CAD build for the part. Positions are in the model's coordinates, mm. Face numbers are marked on the shaded views. A direction names the side the tool comes from. Coordinates: 2 decimals unless noted, no trailing zeros. Write each loop counter-clockwise with the first axis right and the second up, starting at its lowest first coordinate (ties: lowest second). Pieces come first, ordered by that corner, then holes. Notation, with made-up numbers: (5, 69.5) -> (22, 69.5) arc R34 cw to (22, 106.5) -> close; hole circle Ø4 at (87, 17.25). An arc over 180 degrees is marked (long way). Answer as CSV lines item,"result". Start each with the question number.
```python
from build123d import *

# Parameters (mm, degrees)
SKETCH1_W                      = 114.3
SKETCH1_H                      = 139.7
BOSS_EXTRUDE1_DEPTH            = 31.836483884
SKETCH2_W                      = 109.4232
SKETCH2_H                      = 29.474283884
CUT_EXTRUDE1_DEPTH             = 203.397374705
M4_CLEARANCE_HOLE1_D           = 4.7625
M4_CLEARANCE_HOLE1_DEPTH       = 31.836483884
M3_CLEARANCE_HOLE1_D           = 3.59918
M2_CLEARANCE_HOLE1_D           = 2.286
M2_CLEARANCE_HOLE1_DEPTH       = 31.836483884
M4_CLEARANCE_HOLE2_D           = 4.7625
F_3_1_3_1_DIAMETER_HOLE1_D     = 3.1
M4_CLEARANCE_HOLE3_D           = 4.7625
M4_CLEARANCE_HOLE3_DEPTH       = 2.3622
F_3_1_3_1_DIAMETER_HOLE2_D     = 3.1
F_3_1_3_1_DIAMETER_HOLE2_DEPTH = 2.3622
FILLET1_R                      = 0.7366
FILLET2_R                      = 3.175


with BuildPart() as part:
    # Sketch1 → Boss-Extrude1 (new body)
    with BuildSketch(Plane.XZ.offset(31.836483884)):
        with Locations((85.8012, -50.8)):
            Rectangle(SKETCH1_W, SKETCH1_H)
    extrude(amount=-BOSS_EXTRUDE1_DEPTH)

    # Sketch2 → Cut-Extrude1 (cut, through all)
    with BuildSketch(Plane(origin=(0, 0, -120.65), x_dir=(-1, 0, 0), z_dir=(0, 0, -1))):
        with Locations((-85.725, -17.099341942)):
            Rectangle(SKETCH2_W, SKETCH2_H)
    extrude(amount=-CUT_EXTRUDE1_DEPTH, mode=Mode.SUBTRACT)

    # M4 Clearance Hole1
    with Locations(Plane(origin=(0, 0, 0), x_dir=(1, 0, 0), z_dir=(0, 1, 0))):
        with Locations((117.475, 95.25), (53.975, 51.246745007), (117.475, 51.246745007), (53.975, 95.25)):
            Hole(M4_CLEARANCE_HOLE1_D / 2, depth=M4_CLEARANCE_HOLE1_DEPTH)

    # M3 Clearance Hole1 (through all)
    with Locations(Plane(origin=(0, 0, 0), x_dir=(1, 0, 0), z_dir=(0, 1, 0))):
        with Locations((104.4702, -12.7), (53.74894, 28.51658), (105.08488, 33.24352), (53.91894, 1.777120394)):
            Hole(M3_CLEARANCE_HOLE1_D / 2)

    # M2 Clearance Hole1
    with Locations(Plane(origin=(0, 0, 0), x_dir=(1, 0, 0), z_dir=(0, 1, 0))):
        with Locations((92.456, 107.95), (78.994, 107.95), (78.994, -12.7), (92.456, -12.7)):
            Hole(M2_CLEARANCE_HOLE1_D / 2, depth=M2_CLEARANCE_HOLE1_DEPTH)

    # M4 Clearance Hole2 (through all)
    with Locations(Plane(origin=(142.9512, 0, 0), x_dir=(0, 0, -1), z_dir=(1, 0, 0))):
        with Locations((12.7, -19.136483884), (-12.7, -19.136483884), (0, -19.136483884), (88.9, -19.136483884), (101.6, -19.136483884), (114.3, -19.136483884)):
            Hole(M4_CLEARANCE_HOLE2_D / 2)

    # Ø3.1 (3.1) Diameter Hole1 (through all)
    with Locations(Plane(origin=(142.9512, 0, 0), x_dir=(0, 0, -1), z_dir=(1, 0, 0))):
        with Locations((47.09318, -27.181483884), (87.75, -27.181483884), (47.09318, -10.881483884), (87.77636, -10.881483884), (6.41, -10.881483884), (6.41, -27.181483884)):
            Hole(F_3_1_3_1_DIAMETER_HOLE1_D / 2)

    # M4 Clearance Hole3
    with Locations(Plane(origin=(31.0134, 0, 0), x_dir=(0, 0, -1), z_dir=(1, 0, 0))):
        with Locations((12.7, -19.136483884), (-12.7, -19.136483884), (0, -19.136483884)):
            Hole(M4_CLEARANCE_HOLE3_D / 2, depth=M4_CLEARANCE_HOLE3_DEPTH)

    # Ø3.1 (3.1) Diameter Hole2
    with Locations(Plane(origin=(31.0134, 0, 0), x_dir=(0, 0, -1), z_dir=(1, 0, 0))):
        with Locations((47.05, -27.181483884), (87.75, -27.181483884), (47.05, -10.881483884), (87.75, -10.881483884)):
            Hole(F_3_1_3_1_DIAMETER_HOLE2_D / 2, depth=F_3_1_3_1_DIAMETER_HOLE2_DEPTH)

    # Fillet1
    fillet1_edges = [part.edges().sort_by_distance(p)[0] for p in [
        (140.4366, -2.3622, -50.8),
        (31.0134, -2.3622, -50.8),
    ]]
    fillet(fillet1_edges, radius=FILLET1_R)

    # Fillet2
    fillet2_edges = [part.edges().sort_by_distance(p)[0] for p in [
        (28.6512, 0, -50.8),
        (142.9512, 0, -50.8),
    ]]
    fillet(fillet2_edges, radius=FILLET2_R)


solid = part.part
```
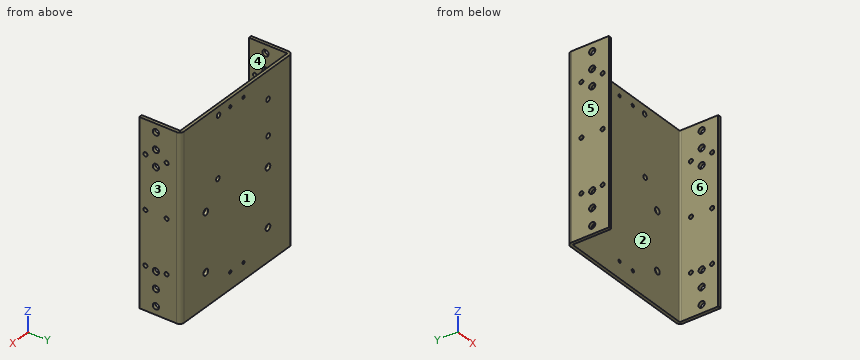
1. Tool access for the marked faces 1 and 2: list every direction of +Z, -Z, +X, -X, +Y, -Y with a clear straight run to the whole face (end or side of a thin tool).
2. Wall check: line 1 (X direction, y = -6.5, z = -24.5); line 2 (X direction, y = -1, z = 12); line 3 (Y direction, x = 75.5, z = -108). Give the ranges that are in metal, low to high.
3. Cut at B-B (z = -114.3). Give the cut face in (x, y) (3 decimals).
4. Cut at D-D (x = 131). Give the cut face in (y, z).
5. Mould opens along X. For the marked faces 3, 4, 5 and 6 say: pulls with the +X half, pulls with the -X half, needs draft (parallel to the pull), parting line crosses it, or undercut.
6. Cut at A-A (y = -6). Give the cut face in (x, z).
7. Flat gauge pins, fed straight in: P1, Ø7.5, axis at x = 53.98, z = -51.25, coming from the -Y side; P2, Ø4.5, axis at x = 117.475, z = -95.25, coming from the +Y side. Where does each tip first touch, or does it go through?
8. Cut at C-C (z = -13.5). Give the cut face in (x, y) (3 decimals).
Geometry check:
1,face 1,"+Z, -Z, +X, -X, +Y"
1,face 2,"+Z, -Z, -Y"
2,line 1,"28.65 to 31.01, 140.44 to 142.95"
2,line 2,"29.51 to 78.09, 79.9 to 91.55, 93.36 to 102.81, 106.13 to 142.09"
2,line 3,"-2.36 to 0"
3,outline,"(28.651, -31.836) -> (31.013, -31.836) -> (31.013, -21.518) -> (28.651, -21.518) -> close; (28.651, -16.755) -> (31.013, -16.755) -> (31.013, -3.099) arc R0.737 cw to (31.75, -2.362) -> (139.7, -2.362) arc R0.737 cw to (140.437, -3.099) -> (140.437, -16.755) -> (142.951, -16.755) -> (142.951, -3.175) arc R3.175 ccw to (139.776, 0) -> (31.826, 0) arc R3.175 ccw to (28.651, -3.175) -> close; (140.437, -31.836) -> (142.951, -31.836) -> (142.951, -21.518) -> (140.437, -21.518) -> close"
4,outline,"(-2.36, -120.65) -> (0, -120.65) -> (0, 19.05) -> (-2.36, 19.05) -> close"
5,face 3,"pulls with the +X half"
5,face 4,"undercut"
5,face 5,"pulls with the -X half"
5,face 6,"undercut"
6,outline,"(28.65, -120.65) -> (31.01, -120.65) -> (31.01, 19.05) -> (28.65, 19.05) -> close; (140.44, -120.65) -> (142.95, -120.65) -> (142.95, 19.05) -> (140.44, 19.05) -> close"
7,P1,"y = -2.36"
7,P2,"through"
8,outline,"(28.651, -31.836) -> (31.013, -31.836) -> (31.013, -21.379) -> (28.651, -21.379) -> close; (28.651, -16.894) -> (31.013, -16.894) -> (31.013, -3.099) arc R0.737 cw to (31.75, -2.362) -> (139.7, -2.362) arc R0.737 cw to (140.437, -3.099) -> (140.437, -16.894) -> (142.951, -16.894) -> (142.951, -3.175) arc R3.175 ccw to (139.776, 0) -> (31.826, 0) arc R3.175 ccw to (28.651, -3.175) -> close; (140.437, -31.836) -> (142.951, -31.836) -> (142.951, -21.379) -> (140.437, -21.379) -> close"
